Autodesk Fusion 360 part; units mm, degrees
sketch "Sketch1" plane through (0, 0, 0) normal (0, 1, 0) x (1, 0, 0)
  line L0 (29, 0) -> (40, 0)
  line L1 (40, 0) -> (40, -55)
  line L2 (40, -55) -> (20, -55)
  line L3 (0, -55) -> (0, -32)
  line L4 (0, -70) -> (0, -85)
  line L5 (0, -35) -> (0, -32)
  line L6 (-29, 0) -> (-40, 0)
  line L7 (-40, 0) -> (-40, -55)
  line L8 (-40, -55) -> (-20, -55)
  line L9 (29, 0) -> (29, -32)
  line L10 (29, -32) -> (0, -32)
  line L11 (-29, -32) -> (0, -32)
  line L12 (-29, 0) -> (-29, -32)
  arc A0 (-20, -55) -> (20, -55) centre (0, -55) ccw
  dimension "d1" = 40
  dimension "d2" = 55
  dimension "d3" = 29
  dimension "d4" = 32
  dimension "d5" = 40
extrude "Extrude1" add sketch "Sketch1" along normal mid plane 50
sketch "Sketch2" plane through (0, 0, 32) normal (0, 0, -1) x (1, 0, 0)
  line L0 (-29, 25) -> (-29, -25)
  line L1 (-29, -25) -> (29, -25)
  line L2 (29, -25) -> (29, 25)
  line L3 (29, 25) -> (-29, 25)
  line L4 (40, 15) -> (27, 15)
  line L5 (27, 15) -> (27, -15)
  line L6 (27, -15) -> (40, -15)
  line L7 (40, 15) -> (58, 15)
  line L8 (58, 15) -> (58, -15)
  line L9 (58, -15) -> (40, -15)
  line L10 (0, -35) -> (0, -40)
  line L11 (-58, -15) -> (-40, -15)
  line L12 (-27, -15) -> (-40, -15)
  line L13 (-27, 15) -> (-27, -15)
  line L14 (-40, 15) -> (-27, 15)
  line L15 (-40, 15) -> (-58, 15)
  line L16 (-58, 15) -> (-58, -15)
  dimension "d9" = 13
  dimension "d10" = 30
  dimension "d11" = 18
  dimension "d12" = 30
extrude "Extrude2" add sketch "Sketch2" against normal blind 63 from surface at 32 contours L0 L11 L12 L14 L15 L16 | L2 L4 L6 L7 L8 L9
sketch "Sketch3" plane through (0, 0, 0) normal (0, 1, 0) x (1, 0, 0)
  line L0 (-7.5, -65) -> (-7.5, -55)
  line L1 (7.5, -55) -> (7.5, -65)
  line L2 (-7.5, -55) -> (7.5, -55)
  line L3 (0, -85) -> (0, -96)
  line L4 (-57.9919, -20) -> (-42, -62.9941)
  line L5 (-42, -62.9941) -> (-63.2403, -5.8898)
  line L6 (-63.2403, -5.8898) -> (-39.5238, -69.6512)
  line L7 (-39.5238, -69.6512) -> (-63.2403, -69.6512)
  line L8 (-63.2403, -69.6512) -> (-63.2403, -5.8898)
  line L9 (39.5238, -69.6512) -> (63.2403, -69.6512)
  line L10 (63.2403, -5.8898) -> (39.5238, -69.6512)
  line L11 (63.2403, -69.6512) -> (63.2403, -5.8898)
  line L12 (-7.5, -65) -> (-20, -65)
  line L13 (7.5, -65) -> (20.2492, -65)
  arc A0 (-20, -65) -> (20.2492, -65) centre (0.1246, -54.9377) ccw
  dimension "d24" = 45
extrude "Extrude3" cut sketch "Sketch3" along normal mid plane 70 contours L4 L5 L6 L7 L8 | L9 L10 L11
extrude "Extrude4" cut sketch "Sketch3" against normal blind 30 contours L0 L1 L2 L12 L13 A0
For this review, take the finished solid that the model builds, in its own axes (mm). A direction names the side the tool comes from. Give positions to 0.01 mm unless a question says otherwise; leave off trailing zeros. Loops run counter-clockwise (first coordinate to the right, second up) from the corner with the lowest first, then second, coordinate; pieces in that order, holes last. Notation, with made-up numbers: M 41.25,-29.5 L 52.25,-29.5 A25 cw 52.25,-14.5 Z; hole C 0.5,-6 d7. An arc over 180 degrees is marked long. Answer as a JSON object with one key per item and string values. Group by question number.
Q1. Add section B-B on x = 33.5. Give the boundary of the cut face in (y, z).
Q2. Add section A-A on z = 17. Give the boundary of the cut face in (x, y), and give its area (3 significant figures).
Q3. Mouldability with a two-part tool opening along X and no side actions: class faces 1 (the flat face through (29, 0, 16)), 2 (the flat face through (40, -20, 27)), 3 (the flat face through (35, 0, 63)), 4 (the flat face through (0, 0, 65)) as +X half, -X half, draft (parallel to the pull), parting line (faces both ways), or undercut.
Q4. Insertion check: P1, Ø11, axis at x = 14, y = -17.5, coming from the +Z side; P2, Ø2, axis at y = -4, z = 58, coming from the +X side; P3, Ø10, axis at x = -25, y = 10.5, coming from the +Z side. Each pin has a flat end and moves straight along its axis. Give the tip position at first contact, or say it passes through.
Q5. For probe 1 along X at (y, z) = (0, 14); probe 2 along X at (y, z) = (-1.5, 59.5); probe 3 along X at (y, z) = (-20, 24), list the stretches that pass through material, from the lowest coordinate up. Write a range as [from, to].
Q6. Tool access review of faces 5 (the flat face through (-40, -20, 27)), 6 (the flat face through (-36, 0, 63)), 7 (the flat face through (-29, 0, 16)), 8 (the flat face through (-29, 0, 59)), 9 (the flat face through (0, -12, 55)): name each direction out of +Z, -Z, +X, -X, +Y, -Y from which nothing blocks a thin tool from reaching the whole face with its end or side.
Q7. Add section D-D on z = 53. Give the boundary of the cut face in (x, y), and give its area (3 significant figures).
Checked values:
{
 "1": {"outline": "M -25,0 L 25,0 L 25,55 L 15,55 L 15,63 L -15,63 L -15,55 L -25,55 Z"},
 "2": {"outline": "M -58,-15 L -40,-15 L -40,-25 L -29,-25 L -29,25 L -40,25 L -40,15 L -58,15 Z; M 29,-25 L 40,-25 L 40,-15 L 58,-15 L 58,15 L 40,15 L 40,25 L 29,25 Z", "area": "2,180 mm²"},
 "3": {"face 1": "undercut", "face 2": "+X half", "face 3": "draft", "face 4": "undercut"},
 "4": {"P1": "z = 65", "P2": "x = 44.23", "P3": "z = 63"},
 "5": {"probe 1": "[-58, -29], [29, 58]", "probe 2": "[-43.3, -29], [-19.49, -7.5], [7.5, 19.49], [29, 43.3]", "probe 3": "[-40, -29], [29, 40]"},
 "6": {"face 5": "+Z, -Z, -X, -Y", "face 6": "+Z, -X, +Y, -Y", "face 7": "-Z, +Y, -Y", "face 8": "+Z, +Y, -Y", "face 9": "+Z, -Y"},
 "7": {"outline": "M -45.72,-15 L -40,-15 L -40,-25 L 40,-25 L 40,-15 L 45.72,-15 L 45.72,15 L 40,15 L 40,25 L -40,25 L -40,15 L -45.72,15 Z", "area": "4,340 mm²"}
}
